from build123d import *

# Parameters (mm, degrees)
SKETCH1_R                               = 150
SKETCH1_R_2                             = 15
BOSS_EXTRUDE1_DEPTH                     = 15
CBORE_FOR_M5_HEX_HEAD_BOLT1_D           = 5.3
CBORE_FOR_M5_HEX_HEAD_BOLT1_CBORE_D     = 12.24
CBORE_FOR_M5_HEX_HEAD_BOLT1_CBORE_DEPTH = 3.58
CIRPATTERN1_COUNT                       = 4
SKETCH5_W                               = 17
SKETCH5_H                               = 50
CUT_EXTRUDE1_DEPTH                      = 213.661703181
FILLET1_R                               = 5


with BuildPart() as part:
    # Sketch1 → Boss-Extrude1 (new body)
    with BuildSketch(Plane(origin=(0, 0, 0), x_dir=(1, 0, 0), z_dir=(0, 1, 0))):
        with Locations(Location((0, 0, 0), (0, 0, 270))):
            Circle(SKETCH1_R)
        with Locations(Location((0, 0, 0), (0, 0, 270))):
            Circle(SKETCH1_R_2, mode=Mode.SUBTRACT)
    extrude(amount=BOSS_EXTRUDE1_DEPTH)

    # CBORE for M5 Hex Head Bolt1 (through all)
    with Locations(Plane(origin=(0, 15, -27.5), x_dir=(0, 0, 1), z_dir=(0, 1, 0))):
        with Locations((0, 0)):
            cbore_for_m5_hex_head_bolt1 = CounterBoreHole(CBORE_FOR_M5_HEX_HEAD_BOLT1_D / 2, CBORE_FOR_M5_HEX_HEAD_BOLT1_CBORE_D / 2, CBORE_FOR_M5_HEX_HEAD_BOLT1_CBORE_DEPTH)

    # CirPattern1: CBORE for M5 Hex Head Bolt1 ×4 about axis
    cirpattern1_axis = Axis((0, 0, 0), (0, 1, 0))
    for i in range(1, CIRPATTERN1_COUNT):
        add(cbore_for_m5_hex_head_bolt1.rotate(cirpattern1_axis, i * 360 / CIRPATTERN1_COUNT), mode=Mode.SUBTRACT)

    # Sketch5 → Cut-Extrude1 (cut, through all)
    with BuildSketch(Plane.XZ):
        with Locations((-85, 65)):
            Rectangle(SKETCH5_W, SKETCH5_H)
        with Locations((-85, 0)):
            Rectangle(SKETCH5_W, SKETCH5_H)
        with Locations((-85, -65)):
            Rectangle(SKETCH5_W, SKETCH5_H)
        with Locations((85, 65)):
            Rectangle(SKETCH5_W, SKETCH5_H)
        with Locations((85, 0)):
            Rectangle(SKETCH5_W, SKETCH5_H)
        with Locations((85, -65)):
            Rectangle(SKETCH5_W, SKETCH5_H)
    extrude(amount=-CUT_EXTRUDE1_DEPTH, mode=Mode.SUBTRACT)

    # Fillet1
    fillet1_edges = [part.edges().sort_by_distance(p)[0] for p in [
        (0, 15, -150),
    ]]
    fillet(fillet1_edges, radius=FILLET1_R)


solid = part.part
Part model, mm, in its own coordinate system. A direction names the side the tool comes from. Round coordinates to 2 decimals unless told otherwise and drop trailing zeros. Put each result on its own line as item: value.
Q1. Band-saw the part on A-A (y = 6). State how many separate pieces and enclosed holes the cut face has, and give its area (3 significant figures).
From the geometry:
separate pieces: 1
enclosed holes: 11
area: 64,800 mm2
Q2. Pin check, flat tips, straight feed: pin 1 Ø4 at (x, z) = (-27.5, 0) entering from -Y; pin 2 Ø7.5 at (y, z) = (5, 68.5) entering from -X (3 decimals); pin 3 Ø6 at (x, z) = (28.5, -3) entering from +Y; pin 4 Ø4.5 at (y, z) = (4.5, 8.5) entering from +X. Stop position of each tip, or through.
From the geometry:
pin 1: passes through
pin 2: stops at x = -135.305
pin 3: stops at y = 15
pin 4: stops at x = 149.87
Q3. Pull direction Z, two halves, no side cores. Call faces 3 (the face through (-91.273, 4.93, -119.035)), 4 (the face through (85, 7, 90)), 5 (the face through (34, 15, -2)): pulls with the +Z half, pulls with the -Z half, needs draft (parallel to the pull), parting line crosses it, or undercut.
From the geometry:
face 3: parting line crosses it
face 4: undercut
face 5: needs draft
Q4. Wall check: line 1 (Y direction, x = 124.5, z = -74.5); line 2 (X direction, y = 12.5, z = -52); line 3 (Z direction, x = 11, y = 12.75). Give the ranges that are in metal, low to high. Write a range as [from, to].
From the geometry:
line 1: y = [0, 15]
line 2: x = [-139.98, -93.5], [-76.5, 76.5], [93.5, 139.98]
line 3: z = [-148.77, -10.2], [10.2, 148.77]
Q5. Tool access for faces 1 (the face through (-26, 11.42, 3)), 2 (the face through (85, 7, -90)): list every direction of +Z, -Z, +X, -X, +Y, -Y with a clear straight run to the whole face (end or side of a thin tool).
From the geometry:
face 1: +Y
face 2: +Y, -Y
